Part model, mm, in its own coordinate system. A direction names the side the tool comes from. Coordinates: 2 decimals unless noted, no trailing zeros. Loops run counter-clockwise (first coordinate to the right, second up) from the corner with the lowest first, then second, coordinate; pieces in that order, holes last. Notation, with made-up numbers: (89, 78.25) - (136, 78.25) arc R11 ccw to (136, 99.25) - close; hole circle Ø1 at (-20.75, 17.5). An arc over 180 degrees is marked (long way). Use a Markdown table: item, result. Add a question column.
1. Pull direction X, two halves, no side cores. Call faces 1 (the flat face through (-4, 54, 71)), 2 (the flat face through (0, 47, 60)), 3 (the flat face through (30, 60, 56)), 4 (the flat face through (-23, 40, 56)): pulls with the +X half, pulls with the -X half, needs draft (parallel to the pull), parting line crosses it, or undercut.
2. Band-saw the part on D-D, the plane y = 33. Give the cut face in (x, z), plus the area to 3 significant figures.
3. Band-saw the part on B-B, the plane x = -1.5. Give the cut face in (y, z), plus the area to 3 significant figures.
4. 3-axis set-ups, long thin cutter, end or side, ignore diameter. For faces 5 (the flat face through (4, 54, 71)), 6 (the flat face through (-15, 20, 40)), 7 (the flat face through (15, 20, 42)): which of +Z, -Z, +X, -X, +Y, -Y reach the whole face in a straight line?
5. Wall check: probe 1 along X at (y, z) = (43, 82); probe 2 along Y at (x, z) = (22, 47); probe 3 along Z at (x, y) = (14, 35). Give the ranges that are in metal, low to high. Write a range as [from, to].
6. Band-saw the part on A-A, the plane z = 69. Give the cut face in (x, y), plus the area to 3 significant figures.
7. Band-saw the part on C-C, the plane z = 38.5. Give the cut face in (x, y).
8. Drop flat-ended pins along their axis: pin 1 (12 mm diameter, centred on x = 19.5, z = 67.5, fed in from -Y); pin 2 (4 mm diameter, centred on x = -1.5, y = 50.5, fed in from +Z); pin 3 (8 mm diameter, centred on x = 3.5, z = 77.5, fed in from -Y). Give the stop position or say it passes through.
from build123d import *

# Parameters (mm, degrees)
PAD_DEPTH       = 30
SKETCH002_W     = 40
SKETCH002_H     = 90
POCKET_DEPTH    = 15
SKETCH003_W     = 40
SKETCH003_H     = 90
POCKET001_DEPTH = 15
SKETCH004_W     = 30
SKETCH004_H     = 8
POCKET002_DEPTH = 80.001


with BuildPart() as part:
    # Sketch → Pad (new body, symmetric)
    with BuildSketch(Plane.YZ):
        with BuildLine():
            ThreePointArc((70, 0), (40, 30), (10, 0))
            Line((10, 0), (0, 0))
            Line((0, 0), (0, 50))
            Line((0, 50), (50, 90))
            Line((50, 90), (80, 90))
            Line((80, 90), (80, 0))
            Line((80, 0), (70, 0))
        make_face()
    extrude(amount=PAD_DEPTH, both=True)

    # Sketch002 (on Face9 of Pad) → Pocket (cut)
    with BuildSketch(Plane.YZ.offset(30)):
        with Locations((20, 45)):
            Rectangle(SKETCH002_W, SKETCH002_H)
    extrude(amount=-POCKET_DEPTH, mode=Mode.SUBTRACT)

    # Sketch003 (on Face2 of Pocket) → Pocket001 (cut)
    with BuildSketch(Plane(origin=(-30, 0, 0), x_dir=(0, 1, 0), z_dir=(-1, 0, 0))):
        with Locations((20, -45)):
            Rectangle(SKETCH003_W, SKETCH003_H)
    extrude(amount=-POCKET001_DEPTH, mode=Mode.SUBTRACT)

    # Sketch004 (on Face10 of Pocket001) → Pocket002 (cut, through all)
    with BuildSketch(Plane.ZX.offset(80)):
        with Locations((75, 0)):
            Rectangle(SKETCH004_W, SKETCH004_H)
    extrude(amount=-POCKET002_DEPTH, mode=Mode.SUBTRACT)


solid = part.part
Geometry check:
| question | item | result |
|---|---|---|
| 1 | face 1 | undercut |
| 1 | face 2 | undercut |
| 1 | face 3 | pulls with the +X half |
| 1 | face 4 | needs draft |
| 2 | outline | (-15, 29.17) - (15, 29.17) - (15, 76.4) - (4, 76.4) - (4, 60) - (-4, 60) - (-4, 76.4) - (-15, 76.4) - close |
| 2 | area | 1,290 mm^2 |
| 3 | outline | (0, 0) - (10, 0) arc R30 cw to (70, 0) - (80, 0) - (80, 60) - (12.5, 60) - (0, 50) - close |
| 3 | area | 3,320 mm^2 |
| 4 | face 5 | +Z, +Y, -Y |
| 4 | face 6 | +Z, -Z, -X, -Y |
| 4 | face 7 | +Z, -Z, +X, -Y |
| 5 | probe 1 | x = [-30, -4], [4, 30] |
| 5 | probe 2 | y = [40, 80] |
| 5 | probe 3 | z = [29.58, 78] |
| 6 | outline | (-30, 40) - (-15, 40) - (-15, 23.75) - (-4, 23.75) - (-4, 80) - (-30, 80) - close; (4, 23.75) - (15, 23.75) - (15, 40) - (30, 40) - (30, 80) - (4, 80) - close |
| 6 | area | 2,440 mm^2 |
| 7 | outline | (-30, 40) - (-15, 40) - (-15, 0) - (15, 0) - (15, 40) - (30, 40) - (30, 80) - (-30, 80) - close |
| 8 | pin 1 | stops at y = 16.91 |
| 8 | pin 2 | stops at z = 60 |
| 8 | pin 3 | stops at y = 29.41 |
